```python
from build123d import *

# Parameters (mm, degrees)
ESBO_O1_R                = 1.5
ESBO_O1_R_2              = 2
RESSALTO_EXTRUS_O1_DEPTH = 1.7
ESBO_O2_W                = 4.3
ESBO_O2_H                = 5.17
RESSALTO_EXTRUS_O2_DEPTH = 0.9
CHANFRO1_SIZE            = 0.7


with BuildPart() as part:
    # Esboço1 → Ressalto-extrusão1 (new body)
    with BuildSketch(Plane(origin=(0, 0, 0), x_dir=(1, 0, 0), z_dir=(0, 1, 0))):
        with BuildLine():
            Line((-23.75, 45.625), (23.75, 45.625))
            Line((23.75, 45.625), (23.75, -45.625))
            ThreePointArc((23.75, -45.625), (0, -69.375), (-23.75, -45.625))
            Line((-23.75, -45.625), (-23.75, 45.625))
        make_face()
        with Locations(Location((-21.25, 43.125, 0), (0, 0, 270))):
            Circle(ESBO_O1_R, mode=Mode.SUBTRACT)
        with Locations(Location((21.25, 43.125, 0), (0, 0, 90))):
            Circle(ESBO_O1_R, mode=Mode.SUBTRACT)
        with Locations(Location((17.320508076, -35.625, 0), (0, 0, 270))):
            Circle(ESBO_O1_R_2, mode=Mode.SUBTRACT)
        with Locations(Location((17.320508076, -55.625, 0), (0, 0, 270))):
            Circle(ESBO_O1_R_2, mode=Mode.SUBTRACT)
        with Locations(Location((-17.320508076, -55.625, 0), (0, 0, 270))):
            Circle(ESBO_O1_R_2, mode=Mode.SUBTRACT)
        with Locations(Location((-17.320508076, -35.625, 0), (0, 0, 270))):
            Circle(ESBO_O1_R_2, mode=Mode.SUBTRACT)
    extrude(amount=RESSALTO_EXTRUS_O1_DEPTH)

    # Esboço2 → Ressalto-extrusão2 (add)
    with BuildSketch(Plane.XZ):
        with Locations((0, 46.25)):
            Rectangle(ESBO_O2_W, ESBO_O2_H)
    extrude(amount=RESSALTO_EXTRUS_O2_DEPTH)

    # Chanfro1
    chanfro1_edges = [part.edges().sort_by_distance(p)[0] for p in [
        (2.15, 0, 46.25),
        (-2.15, 0, 46.25),
    ]]
    chamfer(chanfro1_edges, length=CHANFRO1_SIZE)


solid = part.part
```
Build history of the part. All positions in model axes, mm. Round coordinates to 2 decimals unless told otherwise and drop trailing zeros. Order: outer loops, then holes, each group sorted by start corner. A loop starts at its lowest first (then second) coordinate and runs counter-clockwise, first axis right, second up. Notation, with made-up numbers: (49.5, 24.25) - (81.5, 24.25) arc R34 ccw to (81.5, 63.25) - close; hole circle Ø8 at (80, 36). An arc over 180 degrees is marked (long way). Use a Markdown table: item, result.
1) Pull direction Z, two halves, no side cores. Call faces 1 (the face through (0.52, 0.84, 69.37)), 2 (the face through (0, 0, 11)), 3 (the face through (15.546, 0.838, 36.548)): pulls with the +Z half, pulls with the -Z half, needs draft (parallel to the pull), parting line crosses it, or undercut.
Recorded:
| item | result |
|---|---|
| face 1 | pulls with the +Z half |
| face 2 | needs draft |
| face 3 | undercut |
2) Saw through at B-B on y = 1.25. Give the number of separate pieces and of enclosed holes in the cut face, and give its area (3 significant figures).
Recorded:
| item | result |
|---|---|
| separate pieces | 1 |
| enclosed holes | 6 |
| area | 5,160 mm² |
3) Flat gauge pins, fed straight in: pin 1 Ø0.7 at (x, y) = (-0.5, -0.5) entering from -Z (3 decimals); pin 2 Ø8 at (x, z) = (17, 47) entering from -Y. Where does each tip first touch, or does it go through?
Recorded:
| item | result |
|---|---|
| pin 1 | stops at z = 43.665 |
| pin 2 | stops at y = 0 |
4) Saw through at C-C on x = 21.25. Write the cut outline in (y, z) (3 decimals).
Recorded:
| item | result |
|---|---|
| outline | (0, -45.625) - (1.7, -45.625) - (1.7, -44.625) - (0, -44.625) - close; (0, -41.625) - (1.7, -41.625) - (1.7, 56.232) - (0, 56.232) - close |
5) Wall check: L1, parallel to Z at x = -16.5, y = 0.9 (3 decimals); L2, parallel to Z at x = 19, y = 0.8 (3 decimals); L3, parallel to Y at x = 16, z = 15.5. Give the ranges that are in metal, low to high.
Recorded:
| item | result |
|---|---|
| L1 | z = -45.625 to 33.801, 37.449 to 53.801, 57.449 to 62.708 |
| L2 | z = -45.625 to 34.539, 36.711 to 54.539, 56.711 to 59.875 |
| L3 | y = 0 to 1.7 |
6) Saw through at A-A on x = 0. Write the cut outline in (y, z) (3 decimals), and give its area (3 significant figures).
Recorded:
| item | result |
|---|---|
| outline | (-0.9, 43.665) - (0, 43.665) - (0, -45.625) - (1.7, -45.625) - (1.7, 69.375) - (0, 69.375) - (0, 48.835) - (-0.9, 48.835) - close |
| area | 200 mm² |
7) Saw through at D-D on z = -16. Write the cut outline in (x, y), and give its area (4 significant figures).
Recorded:
| item | result |
|---|---|
| outline | (-23.75, 0) - (23.75, 0) - (23.75, 1.7) - (-23.75, 1.7) - close |
| area | 80.75 mm² |
